from build123d import *

# Parameters (mm, degrees)
F0_W      = 100
F0_H      = 35
F1_DEPTH  = 18
F2_R      = 12.7
F3_DEPTH  = 19
F4_R      = 25
F4_R_2    = 12.7
F5_DEPTH  = 5.5
F6_R      = 2.5
F7_DEPTH  = 3
F8_W      = 100
F8_H      = 57
F8_H_2    = 18
F9_DEPTH  = 12
F11_DEPTH = 50
F13_D     = 12
F13_DEPTH = 12
F14_W     = 15
F14_H     = 18
F15_DEPTH = 35
F17_W     = 150.604561
F17_H     = 102.203328
F18_DEPTH = 94
F19_R     = 12.5
F20_DEPTH = 25


with BuildPart() as f1:
    # F0 (on Top) → F1 (new body)
    with BuildSketch(Plane.XY):
        Rectangle(F0_W, F0_H)
    extrude(amount=-F1_DEPTH)

    # F2 (on face) → F3 (join)
    with BuildSketch(Plane.XY):
        Circle(F2_R)
    extrude(amount=F3_DEPTH)

    # F4 (on face) → F5 (join)
    with BuildSketch(Plane.XY.offset(19)):
        Circle(F4_R)
        Circle(F4_R_2, mode=Mode.SUBTRACT)
        Circle(F4_R_2)
    extrude(amount=F5_DEPTH)

    # F6 (on face) → F7 (join)
    with BuildSketch(Plane.XY.offset(24.5)):
        Circle(F6_R)
    extrude(amount=F7_DEPTH)

    # F8 (on face) → F9 (join)
    with BuildSketch(Plane.XZ.offset(17.5)):
        with Locations((0, -46.5)):
            Rectangle(F8_W, F8_H)
        with Locations((0, -9)):
            Rectangle(F8_W, F8_H_2)
    extrude(amount=F9_DEPTH)

    # F10 (on face) → F11 (cut)
    with BuildSketch(Plane.XZ.offset(29.5)):
        Polygon((-37.5, -50), (-37.5, 0), (-50, 0), (-50, -75), (50, -75), (50, 0), (37.5, 0), (37.5, -50), align=None)
    extrude(amount=-F11_DEPTH, mode=Mode.SUBTRACT)

    # F13
    with Locations(Plane(origin=(0, -17.5, 0), x_dir=(-1, 0, 0), z_dir=(0, 1, 0))):
        with Locations((-22.5, -35), (22.5, -35)):
            Hole(F13_D / 2, depth=F13_DEPTH)

    # F14 (on face) → F15 (cut)
    with BuildSketch(Plane(origin=(0, 17.5, 0), x_dir=(-1, 0, 0), z_dir=(0, 1, 0))):
        with Locations((-30, -9)):
            Rectangle(F14_W, F14_H)
        with Locations((30, -9)):
            Rectangle(F14_W, F14_H)
    extrude(amount=-F15_DEPTH, mode=Mode.SUBTRACT)

    # F17 (on offset) → F18 (cut)
    with BuildSketch(Plane(origin=(0, -23.5, -75), x_dir=(1, 0, 0), z_dir=(0, 0, -1))):
        with Locations((5.335175, 0.654457)):
            Rectangle(F17_W, F17_H)
    extrude(amount=-F18_DEPTH, mode=Mode.SUBTRACT)

    # F19 (on face) → F20 (cut)
    with BuildSketch(Plane(origin=(0, 0, 19), x_dir=(1, 0, 0), z_dir=(0, 0, -1))):
        Circle(F19_R)
    extrude(amount=-F20_DEPTH, mode=Mode.SUBTRACT)


solid = f1.part
Design review of the part built by this model. Coordinates are the model's own, in mm. Coordinates: 2 decimals unless noted, no trailing zeros. Write each loop counter-clockwise with the first axis right and the second up, starting at its lowest first coordinate (ties: lowest second). Pieces come first, ordered by that corner, then holes. Notation, with made-up numbers: (-39, -39) - (3, -39) arc R24 ccw to (3, -20) - close; hole circle Ø5 at (-20, 5). An arc over 180 degrees is marked (long way). One line per item, written item: value.
1) Add section D-D (x = -14). State the section outline as (y, z) points.
Answer sheet:
outline: (-20.71, 19) - (20.71, 19) - (20.71, 24.5) - (-20.71, 24.5) - close
2) To check wall thickness, follow probe 1 along Y at (x, z) = (0, 20.6); probe 2 along X at (y, z) = (-0.5, 22.3) (3 decimals); probe 3 along Y at (x, z) = (-5.5, 20.75). State the ranges of each line that lie inside material, in increasing order.
Answer sheet:
probe 1: y = -25 to -12.5, 12.5 to 25
probe 2: x = -24.995 to -12.49, 12.49 to 24.995
probe 3: y = -24.39 to -11.22, 11.22 to 24.39
3) Add section A-A (x = 0). State the section outline as (y, z) points, plus the area to 4 significant figures.
Answer sheet:
outline: (-25, 19) - (-12.5, 19) - (-12.5, 24.5) - (-25, 24.5) - close; (12.5, 19) - (25, 19) - (25, 24.5) - (12.5, 24.5) - close
area: 137.5 mm2
4) Add section C-C (z = 21.15). State the section outline as (x, y) points.
Answer sheet:
outline: circle Ø50 at (0, 0); hole circle Ø25 at (0, 0)
5) Mouldability with a two-part tool opening along Y and no side actions: class faces 1 (the face through (11.923, -3.755, 21.712)), 2 (the face through (-11.5, 5.9, 24.5)), 3 (the face through (23.846, 7.509, 21.712)) as +Y half, -Y half, draft (parallel to the pull), parting line (faces both ways), or undercut.
Answer sheet:
face 1: undercut
face 2: draft
face 3: parting line
